Autodesk Inventor part; units mm, degrees
ref_plane "YZ Plane" through (0, 0, 0) normal (1, 0, 0) x (0, 1, 0)
ref_plane "XZ Plane" through (0, 0, 0) normal (0, 1, 0) x (-1, 0, 0)
ref_plane "XY Plane" through (0, 0, 0) normal (0, 0, 1) x (1, 0, 0)
sketch "Sketch1" plane through (0, 0, 0) normal (0, 1, 0) x (-1, 0, 0)
  circle A0 centre (0, 0) radius 2.5
  circle A1 centre (0, -55) radius 2.5
  arc A2 (0, 8) -> (0, -8) centre (0, 0) ccw
  arc A3 (0, -47) -> (0, -63) centre (0, -55) ccw
  line L0 (0, -63) -> (8, -63)
  line L1 (8, -63) -> (8, -47)
  line L2 (0, -47) -> (8, -47)
  line L3 (0, -8) -> (8, -8)
  line L4 (8, -8) -> (8, 8)
  line L5 (8, 8) -> (0, 8)
  line L6 (0, 2.5) -> (0, -2.5)
  line L7 (0, 0) -> (0, -2.5) construction
  line L8 (0, -8) -> (0, -49.9553) construction
  dimension "d0" = 5
  dimension "d1" = 5
  dimension "d2" = 55
  dimension "d3" = 16
  dimension "d4" = 16
extrude "Extrusion1" add sketch "Sketch1" along normal blind 12.45
sketch "Sketch3" plane through (0, 0, 0) normal (0, -1, 0) x (1, 0, 0)
  circle A0 centre (0, -55) radius 2.5 construction
  arc A1 (0, -63) -> (0, -47) centre (0, -55) ccw construction
  line L0 (0, -47) -> (-8, -47) construction
  line L1 (-8, -47) -> (-8, -63) construction
  line L2 (-8, -63) -> (0, -63) construction
  circle A2 centre (0, 0) radius 2.5 construction
  arc A3 (0, -8) -> (0, 8) centre (0, 0) ccw construction
  line L3 (0, 8) -> (-8, 8) construction
  line L4 (-8, 8) -> (-8, -8) construction
  line L5 (-8, -8) -> (0, -8) construction
  line L6 (-8, -82.5) -> (-68, -82.5)
  line L7 (-68, -82.5) -> (-68, 27.5)
  line L8 (-68, 27.5) -> (-8, 27.5)
  line L9 (-8, 27.5) -> (-8, -82.5)
  line L10 (-68, -27.5) -> (7.195, -27.5) construction
  circle A4 centre (0, 0) radius 2.5 construction
  circle A5 centre (0, -55) radius 2.5 construction
  line L11 (-8, -8) -> (-8, 8)
  dimension "d15" = 27.5
  dimension "d16" = 110
  dimension "d22" = 60
extrude "Extrusion3" add sketch "Sketch3" along normal blind 17.55 and the other way blind 12.45
sketch "Sketch4" plane through (0, 12.45, 0) normal (0, 1, 0) x (1, 0, 0)
  line L0 (-8, 8) -> (-8, 47) construction
  line L1 (-8, 82.5) -> (-68, 82.5) construction
  line L2 (-68, 82.5) -> (-68, -27.5) construction
  line L3 (-68, -27.5) -> (-8, -27.5) construction
  line L4 (-28, -37.155) -> (-28, 112.7267) construction
  line L5 (-28, -22.5) -> (-30.05, -22.5)
  line L6 (-30.05, -22.5) -> (-30.05, 78.5)
  line L7 (-30.05, 78.5) -> (-28, 78.5)
  line L8 (-28, 78.5) -> (-28, -22.5)
  arc A0 (0, -8) -> (0, 8) centre (0, 0) ccw
  line L9 (0, 8) -> (-8, 8)
  line L10 (-8, 47) -> (0, 47)
  arc A1 (0, 47) -> (0, 63) centre (0, 55) ccw
  line L11 (0, 63) -> (-8, 63)
  line L12 (-8, 63) -> (-8, 82.5)
  line L13 (-8, -27.5) -> (-8, -8)
  line L14 (-8, -8) -> (0, -8)
  dimension "d17" = 20
  dimension "d18" = 2.05
  dimension "d19" = 101
  dimension "d20" = 5
revolve "guide_rail_mount" cut sketch "Sketch4" angle 360 about axis through (-28, 12.45, 37.155) along (0, 0, -1)
mirror "Mirror1" about plane through (-68, 0, 27.5) normal (-1, 0, 0)
sketch "Sketch5" plane through (0, 12.45, 0) normal (0, 1, 0) x (1, 0, 0)
  line L0 (-128, 8) -> (-128, 47) construction
  line L1 (-128, 27.5) -> (-8, 27.5) construction
  line L2 (-8, 82.5) -> (-8, -27.5) construction
  line L3 (-8, -27.5) -> (-128, -27.5) construction
  line L4 (-68, -27.5) -> (-68, 82.5) construction
  line L5 (-123, -17.5) -> (-13, -17.5)
  line L6 (-13, -17.5) -> (-13, 72.5)
  line L7 (-13, 72.5) -> (-123, 72.5)
  line L8 (-123, 72.5) -> (-123, -17.5)
  point P0 (0, 0)
  dimension "d23" = 10
  dimension "d26" = 5
extrude "Extrusion4" cut sketch "Sketch5" against normal blind 26
sketch "Sketch6" plane through (0, 12.45, 0) normal (0, 1, 0) x (1, 0, 0)
  line L0 (-68, -27.5) -> (-68, 79.7854) construction
  line L1 (-88, -32.5) -> (-48, -32.5)
  line L2 (-48, -32.5) -> (-48, 32.5)
  line L3 (-48, 32.5) -> (-88, 32.5)
  line L4 (-88, 32.5) -> (-88, -32.5)
  line L5 (-8, -27.5) -> (-128, -27.5)
  line L6 (-105.95, 72.5) -> (-30.05, 72.5)
  line L7 (-68, 72.5) -> (-68, 96.7026) construction
  point P0 (0, 0)
  dimension "d27" = 5
  dimension "d28" = 60
  dimension "d29" = 40
extrude "Extrusion5" cut sketch "Sketch6" against normal through all
sketch "Sketch7" plane through (0, -13.55, 0) normal (0, 1, 0) x (1, 0, 0)
  line L0 (-88, -17.5) -> (-88, 32.5)
  line L1 (-88, -17.5) -> (-96, -17.5)
  line L2 (-96, -17.5) -> (-96, -9.5)
  line L3 (-96, -9.5) -> (-88, -9.5)
  line L4 (-88, -9.5) -> (-88, -17.5)
  line L5 (-88, -17.5) -> (-105.95, -17.5)
  circle A0 centre (-92, -17.5) radius 1.5
  point P0 (0, 0)
  dimension "d32" = 8
  dimension "d33" = 8
  dimension "d36" = 3
extrude "Extrusion6" add sketch "Sketch7" along normal blind 26 contours L1 A0 L2 L3 L0 | L1 A0 picked at (-91.8227, -17.0325)
ref_plane "Work Plane1" through (-68, -17.55, -82.5) normal (-1, 0, 0) x (0, 0, 1)
extrude "Extrusion7" cut sketch "Sketch7" along normal through all both and the other way through all contours A0 L1 | L1 A0
mirror "Mirror2" about plane through (-68, -17.55, -82.5) normal (-1, 0, 0) of "Extrusion6", "Extrusion7"
sketch "Sketch8" plane through (0, 12.45, 0) normal (0, 1, 0) x (1, 0, 0)
  line L0 (-98, 65.1826) -> (-38, 65.1826)
  line L1 (-38, 65.1826) -> (-38, 77.5)
  line L2 (-38, 77.5) -> (-98, 77.5)
  line L3 (-98, 77.5) -> (-98, 65.1826)
  line L4 (-68, -49.5) -> (-68, 104.5) construction
  line L5 (-105.95, 72.5) -> (-30.05, 72.5) construction
  point P0 (0, 0)
  dimension "d39" = 60
  dimension "d40" = 5
extrude "Extrusion8" cut sketch "Sketch8" against normal blind 18
sketch "Sketch9" plane through (0, 0, 8) normal (0, 0, 1) x (1, 0, 0)
  line L0 (0, 0) -> (-8, 0) construction
  line L1 (0, 0) -> (0, 12.45) construction
  line L2 (-8, 12.45) -> (0, 12.45) construction
  line L3 (-8, 0) -> (-8, 12.45) construction
  line L4 (-8, 0) -> (-8, 12.45)
  line L5 (-8, 1.45) -> (23.9687, 1.45)
  line L6 (23.9687, 1.45) -> (23.9687, -24.0835)
  line L7 (23.9687, -24.0835) -> (-8, -24.0835)
  line L8 (-8, -24.0835) -> (-8, 1.45)
  point P0 (0, 0)
  dimension "d43" = 11
extrude "limit-side-to-11mm" cut sketch "Sketch9" against normal through all
mirror "Mirror3" about plane through (-68, -17.55, -82.5) normal (-1, 0, 0) of "limit-side-to-11mm"
properties part number "PRING_piston_holder_half"
Part model, mm, in its own coordinate system. A direction names the side the tool comes from. Coordinates: 2 decimals unless noted, no trailing zeros. Order: outer loops, then holes, each group sorted by start corner. A loop starts at its lowest first (then second) coordinate and runs counter-clockwise, first axis right, second up. Notation, with made-up numbers: M 51,54 L 100,54 A15 ccw 100,58 Z; hole C 81,15 d10. An arc over 180 degrees is marked long. Use a Markdown table: item, result.
(1) Flat gauge pins, fed straight in: pin 1 (1.5 mm diameter, centred on x = -27, z = -40, fed in from +Y); pin 2 (5 mm diameter, centred on x = -135.5, z = -59, fed in from -Y); pin 3 (6.5 mm diameter, centred on x = -136, z = -55, fed in from +Y); pin 4 (2.5 mm diameter, centred on y = 7.5, z = -75, fed in from -X). Where does each tip first touch, or does it go through?
A:
| item | result |
|---|---|
| pin 1 | stops at y = -13.55 |
| pin 2 | stops at y = 1.45 |
| pin 3 | stops at y = 12.45 |
| pin 4 | stops at x = -128 |
(2) Probe L1, parallel to Z at x = -92, y = -2.5; L2, parallel to Z at x = -136, y = 8; L3, parallel to X at y = 11.25, z = -21. List the from-to ranges inside material, lowest first.
A:
| item | result |
|---|---|
| L1 | z = -82.5 to -77.5, 9.5 to 16, 19 to 27.5 |
| L2 | z = -63 to -57.5, -52.5 to -47, -8 to -2.5, 2.5 to 8 |
| L3 | x = -128 to -123, -13 to -8 |
(3) Cut at D-D on x = -6. Write the cut outline in (y, z), then the cut area to 3 significant figures.
A:
| item | result |
|---|---|
| outline | M 1.45,-63 L 12.45,-63 L 12.45,-47 L 1.45,-47 Z; M 1.45,-8 L 12.45,-8 L 12.45,8 L 1.45,8 Z |
| area | 352 mm^2 |
(4) Pull direction X, two halves, no side cores. Call faces 1 (the cylindrical face through (8, 7, 0)), 2 (the cylindrical face through (-28, 10.4, 20)), 3 (the flat face through (-44, -1, 9.5)), 4 (the flat face through (-108, -2, 27.5)): released by +X, released by -X, zero draft, split by the parting line, or undercut.
A:
| item | result |
|---|---|
| face 1 | released by +X |
| face 2 | undercut |
| face 3 | undercut |
| face 4 | zero draft |
(5) Cut at C-C on z = -55. Write the cut outline in (x, y), then the cut area to 3 significant figures.
A:
| item | result |
|---|---|
| outline | M -144,1.45 L -138.5,1.45 L -138.5,12.45 L -144,12.45 Z; M -133.5,1.45 L -128,1.45 L -128,-17.55 L -8,-17.55 L -8,1.45 L -2.5,1.45 L -2.5,12.45 L -13,12.45 L -13,-13.55 L -123,-13.55 L -123,12.45 L -133.5,12.45 Z; M 2.5,1.45 L 8,1.45 L 8,12.45 L 2.5,12.45 Z |
| area | 982 mm^2 |
(6) Cut at B-B on y = -9.5. Write the cut outline in (x, z).
A:
| item | result |
|---|---|
| outline | M -128,-82.5 L -8,-82.5 L -8,27.5 L -48,27.5 L -48,9.5 L -40,9.5 L -40,17.5 L -13,17.5 L -13,-72.5 L -123,-72.5 L -123,17.5 L -96,17.5 L -96,9.5 L -88,9.5 L -88,27.5 L -128,27.5 Z; hole C -92,17.5 d3; hole C -44,17.5 d3 |
(7) Tool access for faces 5 (the flat face through (-92, -1, 9.5)), 6 (the flat face through (-134, 1.45, 2)), 7 (the flat face through (-88, -6, 10)), 8 (the flat face through (-132, 7, -63)): list every direction of +Z, -Z, +X, -X, +Y, -Y with a clear straight run to the whole face (end or side of a thin tool).
A:
| item | result |
|---|---|
| face 5 | +Y |
| face 6 | +Z, -Z, -X, -Y |
| face 7 | +Z, +Y, -Y |
| face 8 | -Z, -X, +Y, -Y |
(8) Cut at A-A on z = 0. Write the cut outline in (x, y).
A:
| item | result |
|---|---|
| outline | M -144,1.45 L -138.5,1.45 L -138.5,12.45 L -144,12.45 Z; M -133.5,1.45 L -128,1.45 L -128,-17.55 L -88,-17.55 L -88,-13.55 L -123,-13.55 L -123,12.45 L -133.5,12.45 Z; M -48,-17.55 L -8,-17.55 L -8,1.45 L -2.5,1.45 L -2.5,12.45 L -13,12.45 L -13,-13.55 L -48,-13.55 Z; M 2.5,1.45 L 8,1.45 L 8,12.45 L 2.5,12.45 Z |
